```python
from build123d import *

# Parameters (mm, degrees)
SKETCH2_W           = 205.74
SKETCH2_H           = 96.52
BOSS_EXTRUDE1_DEPTH = 5.08
SKETCH3_W           = 205.74
SKETCH3_H           = 96.52
SKETCH3_W_2         = 195.58
SKETCH3_H_2         = 86.36
BOSS_EXTRUDE2_DEPTH = 95.25
SKETCH5_W           = 22.490008116
SKETCH5_H           = 8.285792463
CUT_EXTRUDE1_DEPTH  = 95.25


with BuildPart() as part:
    # Sketch2 → Boss-Extrude1 (new body)
    with BuildSketch(Plane(origin=(0, 0, 0), x_dir=(1, 0, 0), z_dir=(0, 1, 0))):
        Rectangle(SKETCH2_W, SKETCH2_H)
    extrude(amount=BOSS_EXTRUDE1_DEPTH)

    # Sketch3 → Boss-Extrude2 (add)
    with BuildSketch(Plane(origin=(0, 5.08, 0), x_dir=(1, 0, 0), z_dir=(0, 1, 0))):
        Rectangle(SKETCH3_W, SKETCH3_H)
        Rectangle(SKETCH3_W_2, SKETCH3_H_2, mode=Mode.SUBTRACT)
    extrude(amount=BOSS_EXTRUDE2_DEPTH)

    # Sketch5 → Cut-Extrude1 (cut)
    with BuildSketch(Plane.XZ):
        with Locations((0, 37.064125217)):
            Rectangle(SKETCH5_W, SKETCH5_H)
    extrude(amount=-CUT_EXTRUDE1_DEPTH, mode=Mode.SUBTRACT)


solid = part.part
```
Input: part model. Units: mm. Frame: model coordinates. A direction names the side the tool comes from. Give positions to 0.01 mm unless a question says otherwise; leave off trailing zeros. Order: outer loops, then holes, each group sorted by start corner. A loop starts at its lowest first (then second) coordinate and runs counter-clockwise, first axis right, second up. Notation, with made-up numbers: (17.25, 3.5) - (30.25, 3.5) arc R19 ccw to (30.25, 23.5) - close; hole circle Ø7 at (31, 70.5). An arc over 180 degrees is marked (long way). Use a Markdown table: item, result.
(1) Section query C-C (z = 18). Output: boundary loops of the cut face in (x, y).
Computed values:
| item | result |
|---|---|
| outline | (-102.87, 0) - (102.87, 0) - (102.87, 100.33) - (97.79, 100.33) - (97.79, 5.08) - (-97.79, 5.08) - (-97.79, 100.33) - (-102.87, 100.33) - close |
(2) Line query: line 1 (X direction, y = 70.5, z = -20.5); line 2 (Z direction, x = 33.5, y = 67); line 3 (Y direction, x = 18, z = -25). Output: solid intervals per line, ascending. Write a range as from..to.
Computed values:
| item | result |
|---|---|
| line 1 | x = -102.87..-97.79, 97.79..102.87 |
| line 2 | z = -48.26..-43.18, 43.18..48.26 |
| line 3 | y = 0..5.08 |
(3) Section query B-B (x = 6.5). Output: boundary loops of the cut face in (y, z), then the cut area to 3 significant figures.
Computed values:
| item | result |
|---|---|
| outline | (0, -48.26) - (100.33, -48.26) - (100.33, -43.18) - (5.08, -43.18) - (5.08, 32.92) - (0, 32.92) - close; (0, 41.21) - (5.08, 41.21) - (5.08, 43.18) - (100.33, 43.18) - (100.33, 48.26) - (0, 48.26) - close |
| area | 1,420 mm2 |
(4) Draft query along Z for faces 4 (the flat face through (-1, 49, 48.26)), 5 (the flat face through (-8, 100.33, 46)), 6 (the flat face through (-1, 5.08, -1)). Return one class per face: released by +Z, released by -Z, zero draft, split by the parting line, or undercut.
Computed values:
| item | result |
|---|---|
| face 4 | released by +Z |
| face 5 | zero draft |
| face 6 | undercut |
(5) Section query A-A (y = 63). Output: boundary loops of the cut face in (x, z), then the cut area to 3 significant figures.
Computed values:
| item | result |
|---|---|
| outline | (-102.87, -48.26) - (102.87, -48.26) - (102.87, 48.26) - (-102.87, 48.26) - close; hole (-97.79, -43.18) - (97.79, -43.18) - (97.79, 43.18) - (-97.79, 43.18) - close |
| area | 2,970 mm2 |
(6) Access query for faces 1 (the flat face through (0, 3, 41.207)), 2 (the flat face through (97.79, 52, 1)), 3 (the flat face through (102.87, 49, 1)). Directions: +Z, -Z, +X, -X, +Y, -Y. A direction counts if a zero-diameter tool reaches every point of the face in a straight line with its end or side. Return the directions, or none.
Computed values:
| item | result |
|---|---|
| face 1 | +Y, -Y |
| face 2 | +Y |
| face 3 | +Z, -Z, +X, +Y, -Y |
